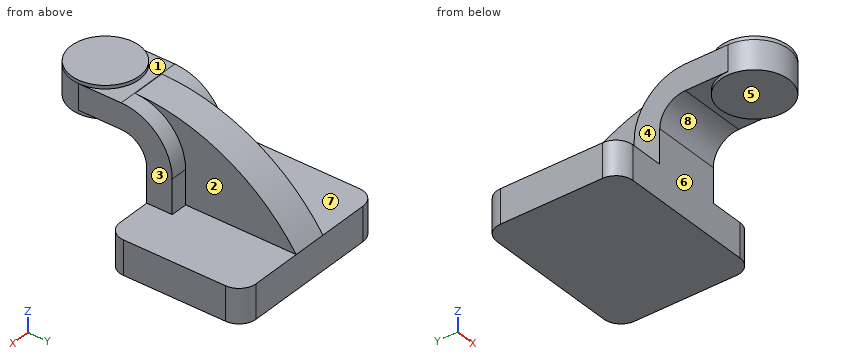
```python
from build123d import *

# Parameters (mm, degrees)
F1_DEPTH      = 25.4
F1_DEPTH_BACK = 25.4
F2_DEPTH      = 63.5
F2_DEPTH_BACK = 63.5
F4_DEPTH      = 2.54
F4_DEPTH_BACK = 21.59
F6_DEPTH      = 12.7
F6_DEPTH_BACK = 12.7
F7_R          = 12.7


with BuildPart() as f1:
    # F0 (on Right) → F1 (new body, two sides)
    with BuildSketch(Plane.YZ) as f1_sk:
        with BuildLine():
            Line((-50.8, 38.1), (-50.8, 12.7))
            Line((-50.8, 12.7), (-31.75, 12.7))
            Line((-31.75, 12.7), (-31.75, 38.1))
            ThreePointArc((-31.75, 38.1), (-42.9092316368, 65.0407683632), (-69.85, 76.2))
            Line((-69.85, 76.2), (-101.6, 76.2))
            Line((-101.6, 76.2), (-101.6, 57.15))
            Line((-101.6, 57.15), (-69.85, 57.15))
            ThreePointArc((-69.85, 57.15), (-56.3796158184, 51.5703841816), (-50.8, 38.1))
        make_face()
    extrude(amount=F1_DEPTH)
    extrude(f1_sk.sketch, amount=-F1_DEPTH_BACK)

    # F0 (on Right) → F2 (join, two sides)
    with BuildSketch(Plane.YZ) as f2_sk:
        Polygon((-50.8, 12.7), (-50.8, -12.7), (50.8, -12.7), (50.8, 12.7), (-31.75, 12.7), align=None)
    extrude(amount=F2_DEPTH)
    extrude(f2_sk.sketch, amount=-F2_DEPTH_BACK)

    # F3 (on face) → F4 (join, two sides)
    with BuildSketch(Plane.XY.offset(76.2)) as f4_sk:
        with BuildLine():
            ThreePointArc((-25.4, -101.6), (0, -127), (25.4, -101.6))
            Line((25.4, -101.6), (-25.4, -101.6))
        make_face()
        with BuildLine():
            Line((-25.4, -101.6), (25.4, -101.6))
            ThreePointArc((25.4, -101.6), (0, -76.2), (-25.4, -101.6))
        make_face()
    extrude(amount=F4_DEPTH)
    extrude(f4_sk.sketch, amount=-F4_DEPTH_BACK)

    # F5 (on Right) → F6 (join, two sides)
    with BuildSketch(Plane.YZ) as f6_sk:
        with BuildLine():
            Line((-31.75, 12.7), (50.8, 12.7))
            ThreePointArc((50.8, 12.7), (-1.5601227987, 59.1215530154), (-69.4199238636, 76.1975725541))
            ThreePointArc((-69.4199238636, 76.1975725541), (-42.7576034578, 64.8882819457), (-31.75, 38.1))
            Line((-31.75, 38.1), (-31.75, 12.7))
        make_face()
    extrude(amount=F6_DEPTH)
    extrude(f6_sk.sketch, amount=-F6_DEPTH_BACK)

    # F7
    f7_edges = [f1.edges().sort_by_distance(p)[0] for p in [
        (-63.5, 50.8, 0),
        (-63.5, -50.8, 0),
        (63.5, -50.8, 0),
        (63.5, 50.8, 0),
    ]]
    fillet(f7_edges, radius=F7_R)


solid = f1.part
```
Read the model definition and answer for the solid it produces. Units are mm, in the model's axes. Face numbers are marked on the shaded views. A direction names the side the tool comes from. Coordinates: 2 decimals unless noted, no trailing zeros. Loops run counter-clockwise (first coordinate to the right, second up) from the corner with the lowest first, then second, coordinate; pieces in that order, holes last.
(1) Flat-ended cylindrical pins translate along their axes: pin 1 Ø15 at (x, z) = (-20.5, 20) entering from -Y; pin 2 Ø5 at (x, z) = (1, 60.5) entering from -Y; pin 3 Ø8 at (x, z) = (7.5, 62) entering from -Y. Find the tip coordinate at first contact, or state that the pin passes through.
Solution:
pin 1: stops at y = -50.8
pin 2: stops at y = -127
pin 3: stops at y = -126.76
(2) The part is cut by section D-D (x = 16). Determine the outline of the cut face in (y, z).
Solution:
outline: (-121.33, 54.61) - (-81.87, 54.61) - (-81.87, 57.15) - (-69.85, 57.15) arc R19.05 cw to (-50.8, 38.1) - (-50.8, -12.7) - (50.8, -12.7) - (50.8, 12.7) - (-31.75, 12.7) - (-31.75, 38.1) arc R38.1 ccw to (-69.85, 76.2) - (-81.87, 76.2) - (-81.87, 78.74) - (-121.33, 78.74) - close
(3) The mould has two halves that part along Y. Classify the marked faces 6, 7 and 8: released by +Y, released by -Y, zero draft, split by the parting line, or undercut.
Solution:
face 6: released by -Y
face 7: zero draft
face 8: undercut
(4) A tool of negligible diameter and unlimited length cuts with its end or side. For the marked faces 1, 2, 3, 4 and 5, from which of +Z, -Z, +X, -X, +Y, -Y can it reach the whole face along a straight path? Write none if from no direction.
Solution:
face 1: +Z, +Y
face 2: +Z, +X, +Y
face 3: +Z, +X, +Y, -Y
face 4: +Z, -X, +Y, -Y
face 5: -Z, +X, -X, -Y
(5) Consider line 1 along Z through (x, y) = (7.5, -115); line 2 along Y through (x, z) = (-51, -4); line 3 along Y through (x, z) = (23, 31). Determine where each line is inside the solid, lowest interval first.
Solution:
line 1: z = 54.61 to 78.74
line 2: y = -50.8 to 50.8
line 3: y = -50.8 to -31.75
(6) The part is cut by section C-C (y = 31). Determine the outline of the cut face in (x, z).
Solution:
outline: (-63.5, -12.7) - (63.5, -12.7) - (63.5, 12.7) - (12.7, 12.7) - (12.7, 35.77) - (-12.7, 35.77) - (-12.7, 12.7) - (-63.5, 12.7) - close
(7) The part is cut by section A-A (z = -0.5). Determine the outline of the cut face in (x, y).
Solution:
outline: (-63.5, -38.1) arc R12.7 ccw to (-50.8, -50.8) - (50.8, -50.8) arc R12.7 ccw to (63.5, -38.1) - (63.5, 38.1) arc R12.7 ccw to (50.8, 50.8) - (-50.8, 50.8) arc R12.7 ccw to (-63.5, 38.1) - close
(8) The part is cut by section B-B (x = 0). Determine the outline of the cut face in (y, z), and give its area (3 significant figures).
Solution:
outline: (-127, 54.61) - (-76.2, 54.61) - (-76.2, 57.15) - (-69.85, 57.15) arc R19.05 cw to (-50.8, 38.1) - (-50.8, -12.7) - (50.8, -12.7) - (50.8, 12.7) arc R147.54 ccw to (-69.42, 76.2) arc R38.1 ccw to (-69.85, 76.2) - (-76.2, 76.2) - (-76.2, 78.74) - (-127, 78.74) - close
area: 8,520 mm2
